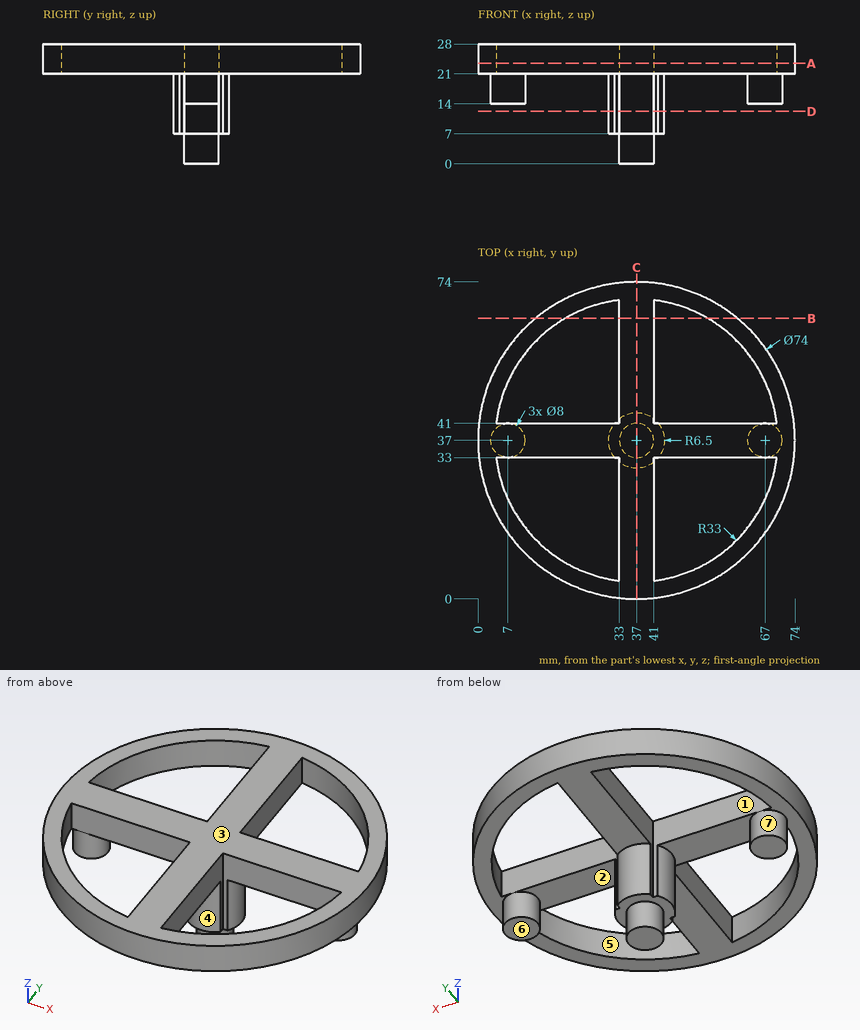
Geometry: see drawing. Coordinates: mm, zero at the bounding-box minimum. A direction names the side the tool comes from. Coordinates: 2 decimals unless noted, no trailing zeros. Loops run counter-clockwise (first coordinate to the right, second up) from the corner with the lowest first, then second, coordinate; pieces in that order, holes last. Notation, with made-up numbers: (-35.75, 2.25) - (10.25, 2.25) arc R30 cw to (10.25, 36.25) - close; hole circle Ø7 at (40, 42). An arc over 180 degrees is marked (long way). Put each result on its own line as item: value. Start each with the question number.
Q1. Pull-direction query (X, two-part tool) for the marked faces 1, 2, 3 and 4; classes: released by +X, released by -X, zero draft, split by the parting line, or undercut.
Q2. Line query: line 1 (Y direction, x = 14.5, z = 26); line 2 (X direction, y = 23.5, z = 21.5). Output: solid intervals per line, ascending.
Q3. Cut plane A-A, the plane z = 23.5. Return loops of the section in (x, y).
Q4. Cut plane B-B, the plane y = 65.5. Return loops of the section in (x, z), and give its area (3 significant figures).
Q5. Cut plane D-D, the plane z = 12.25. Return loops of the section in (x, y).
Q6. Pin query (flat end, axial travel): pin 1 Ø10.5 at (x, z) = (19.5, 13) entering from +Y; pin 2 Ø2.5 at (x, y) = (7.5, 39) entering from -Z; pin 3 Ø4 at (x, z) = (16, 21) entering from -Y; pin 4 Ø10.5 at (y, z) = (55, 20) entering from +X. Return the tip coordinate at first contact, or that it passes through.
Q7. Cut plane C-C, the plane x = 37. Return loops of the section in (y, z), and give its area (3 significant figures).
Q8. Set-up query: the marked faces 5, 6 and 7. Return all of +Z, -Z, +X, -X, +Y, -Y with unobstructed straight access to the full face (end or side cutting, diameter ignored); none if empty.
Filled sheet:
1. face 1: undercut
1. face 2: undercut
1. face 3: zero draft
1. face 4: split by the parting line
2. line 1: 7.63 to 12.86, 33 to 41, 61.14 to 66.37
2. line 2: 2.55 to 6.89, 33 to 41, 67.11 to 71.45
3. outline: circle Ø74 at (37, 37); hole (4.24, 33) arc R33 ccw to (33, 4.24) - (33, 33) - close; hole (4.24, 41) - (33, 41) - (33, 69.76) arc R33 ccw to start; hole (41, 4.24) arc R33 ccw to (69.76, 33) - (41, 33) - close; hole (41, 41) - (69.76, 41) arc R33 ccw to (41, 69.76) - close
4. outline: (13.4, 21) - (20.36, 21) - (20.36, 28) - (13.4, 28) - close; (33, 21) - (41, 21) - (41, 28) - (33, 28) - close; (53.64, 21) - (60.6, 21) - (60.6, 28) - (53.64, 28) - close
4. area: 153 mm²
5. outline: (31.88, 33) - (33, 33) - (33, 31.88) arc R6.5 ccw to (41, 31.88) - (41, 33) - (42.12, 33) arc R6.5 ccw to (42.12, 41) - (41, 41) - (41, 42.12) arc R6.5 ccw to (33, 42.12) - (33, 41) - (31.88, 41) arc R6.5 ccw to start
6. pin 1: through
6. pin 2: z = 14
6. pin 3: y = 5.25
6. pin 4: x = 71.7
7. outline: (0, 21) - (30.5, 21) - (30.5, 7) - (33, 7) - (33, 0) - (41, 0) - (41, 7) - (43.5, 7) - (43.5, 21) - (74, 21) - (74, 28) - (0, 28) - close
7. area: 756 mm²
8. face 5: +Z, -Z
8. face 6: -Z, +X, +Y, -Y
8. face 7: -Z
